Could you check a few things on this model? Use its own coordinates, in mm. A direction names the side the tool comes from. Give positions to 0.01 mm unless a question says otherwise; leave off trailing zeros. Loops run counter-clockwise (first coordinate to the right, second up) from the corner with the lowest first, then second, coordinate; pieces in that order, holes last. Notation, with made-up numbers: (-26.5, 9) - (1.5, 9) arc R15 ccw to (1.5, 31) - close; hole circle Ø1 at (31.25, 5.25). An arc over 180 degrees is marked (long way). One line per item, written item: value. Start each with the question number.
Q1. If I drill on line 1 (Z direction, x = -41, y = 14); line 2 (Y direction, x = -60.5, z = -6); line 3 (X direction, y = 14.5, z = 8), over which ranges is the centre line in solid material (lowest first)? Write a range as from..to.
Q2. I want a section at D-D (x = -22.5). Please give me the cut outline in (y, z).
Q3. For faces 1 (the face through (24.03, 0.63, 14.14)), 2 (the face through (-52, 10, 9.023)), 3 (the face through (23.257, 0.626, -14.084)), 4 (the face through (-52, 10, -7.499)), which set-ups out of +Z, -Z, +X, -X, +Y, -Y let a thin tool reach every point of the face, with its end or its side?
Q4. I want a section at A-A (z = 13.5). Please give me the cut outline in (x, y).
Q5. I want a section at C-C (z = -5). Please give me the cut outline in (x, y), then the cut area to 3 significant figures.
Q6. I want a section at B-B (x = -55). Please give me the cut outline in (y, z).
Q7. I'm going to push flat-ended pins straight in: P1, Ø2, axis at x = 48, z = -7, coming from the -Y side; P2, Ø5, axis at x = -64, y = 10.5, coming from the -Z side; P3, Ø1.7, axis at y = 7.5, z = -8, coming from the +X side; P4, Ø5, axis at x = -43.5, y = 9, coming from the +Z side. Where does each tip first touch, or does it pass through?
```python
from build123d import *

# Parameters (mm, degrees)
BOSS_EXTRUDE1_DEPTH = 1.27
SKETCH5_W           = 50.8
SKETCH5_H           = 1.524
BOSS_EXTRUDE2_DEPTH = 16.764
SKETCH6_R           = 1.27
CUT_EXTRUDE1_DEPTH  = 19.304
FILLET1_R           = 2.54
SKETCH7_R           = 1.27
CUT_EXTRUDE2_DEPTH  = 19.304


with BuildPart() as part:
    # Sketch4 → Boss-Extrude1 (new body)
    with BuildSketch(Plane(origin=(0, 0, 0), x_dir=(1, 0, 0), z_dir=(0, 1, 0))):
        Polygon((87.667304241, 16.16075), (87.093635827, -16.16075), (61.31636847, -16.16075), (-14.309963117, -12.065), (-14.309963117, -16.570075948), (-87.667304241, -15.289618795), (-87.036695722, 15.300626108), (-14.309963117, 16.570075948), (-14.309963117, 12.065), (61.890036883, 16.16075), align=None)
    extrude(amount=BOSS_EXTRUDE1_DEPTH)

    # Sketch5 → Boss-Extrude2 (add)
    with BuildSketch(Plane(origin=(0, 1.27, 0), x_dir=(1, 0, 0), z_dir=(0, 1, 0))):
        with Locations((-53.018825687, -8.260503656)):
            Rectangle(SKETCH5_W, SKETCH5_H)
        with Locations((-53.018825687, 8.260503656)):
            Rectangle(SKETCH5_W, SKETCH5_H)
    extrude(amount=BOSS_EXTRUDE2_DEPTH)

    # Sketch6 → Cut-Extrude1 (cut)
    with BuildSketch(Plane.XY.offset(9.022503656)):
        with Locations((-74.608825687, 15.494)):
            Circle(SKETCH6_R)
    extrude(amount=-CUT_EXTRUDE1_DEPTH, mode=Mode.SUBTRACT)

    # Fillet1
    fillet1_edges = [part.edges().sort_by_distance(p)[0] for p in [
        (-27.618825687, 1.27, -8.260503656),
        (-27.618825687, 18.034, -8.260503656),
        (-78.418825687, 18.034, -8.260503656),
        (-27.618825687, 1.27, 8.260503656),
        (-78.418825687, 18.034, 8.260503656),
        (-27.618825687, 18.034, 8.260503656),
    ]]
    fillet(fillet1_edges, radius=FILLET1_R)

    # Sketch7 → Cut-Extrude2 (cut)
    with BuildSketch(Plane(origin=(0, 1.27, 0), x_dir=(1, 0, 0), z_dir=(0, 1, 0))):
        with Locations(Location((-58.141999981, 0.005503656, 0), (0, 0, 270))):
            Circle(SKETCH7_R)
    extrude(amount=-CUT_EXTRUDE2_DEPTH, mode=Mode.SUBTRACT)


solid = part.part
```
Worked answers:
1. line 1: z = -9.02..-7.5, 7.5..9.02
1. line 2: y = 0..1.27
1. line 3: x = -78.42..-75.4, -73.82..-27.62
2. outline: (0, -16.43) - (1.27, -16.43) - (1.27, 16.43) - (0, 16.43) - close
3. face 1: +Z, +Y, -Y
3. face 2: +Z, +X, -X, +Y
3. face 3: -Z, +Y, -Y
3. face 4: +X, -X, +Y
4. outline: (-87.63, 0) - (-14.31, 0) - (-14.31, 1.27) - (-87.63, 1.27) - close; (12.19, 0) - (87.14, 0) - (87.14, 1.27) - (12.19, 1.27) - close
5. outline: (-87.25, 0) - (87.47, 0) - (87.47, 1.27) - (-87.25, 1.27) - close
5. area: 222 mm²
6. outline: (0, -15.86) - (1.27, -15.86) - (1.27, -9.02) - (18.03, -9.02) - (18.03, -7.5) - (1.27, -7.5) - (1.27, 7.5) - (18.03, 7.5) - (18.03, 9.02) - (1.27, 9.02) - (1.27, 15.86) - (0, 15.86) - close
7. P1: stops at y = 0
7. P2: stops at z = -9.02
7. P3: stops at x = -27.62
7. P4: stops at z = 9.02
